For this review, use the dimensioned drawing (mm, ordinates from the lowest corner) and the shaded views. Coordinates: 2 decimals unless noted, no trailing zeros. Write each loop counter-clockwise with the first axis right and the second up, starting at its lowest first coordinate (ties: lowest second). Pieces come first, ordered by that corner, then holes.
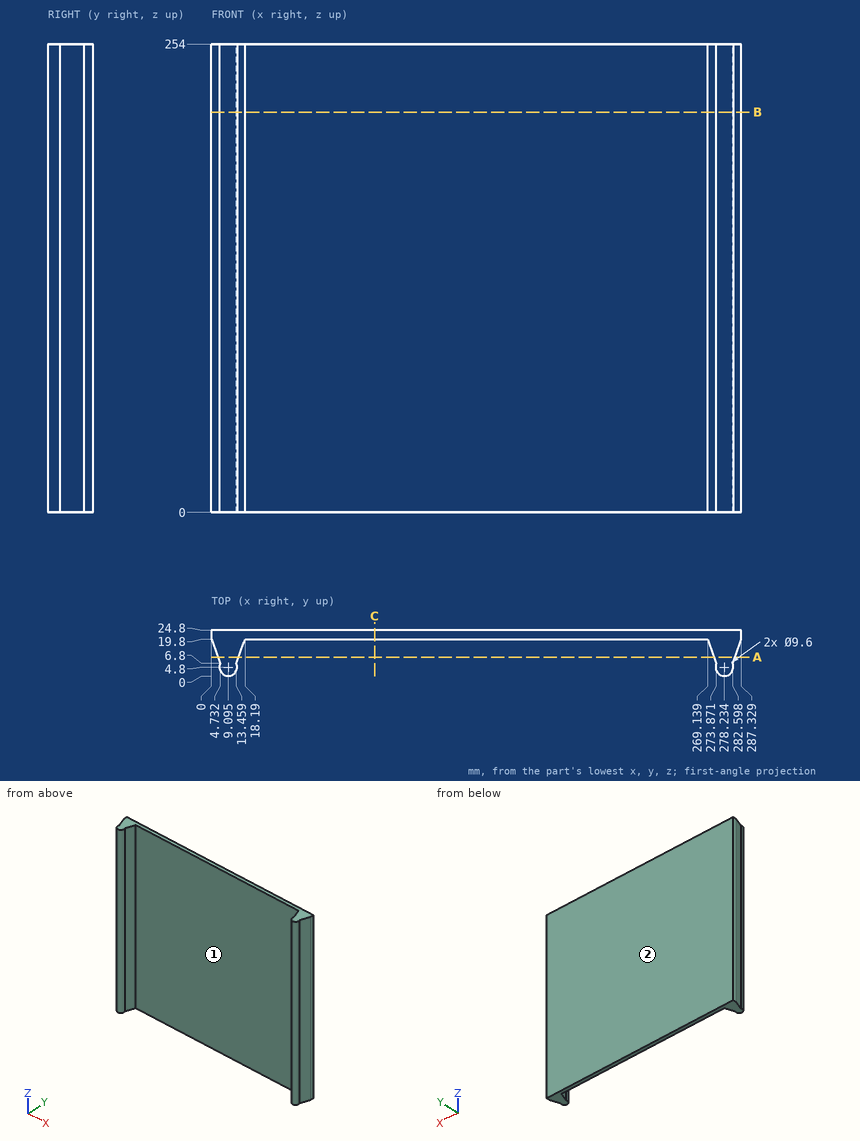
(1) Consider section B-B (z = 217). Give the boundary of the cut face in (x, y) (1 decimal).
(2) Mouldability with a two-part tool opening along X and no side actions: class the marked faces 1 and 2 as +X half, -X half, draft (parallel to the pull), parting line (faces both ways), or undercut.
(3) Consider section C-C (x = 88.5). Give the boundary of the cut face in (y, z), plus the area to 3 significant figures.
(4) Insertion check: pin 1 Ø1.5 at (y, z) = (18.5, 185) entering from +X; pin 2 Ø6 at (y, z) = (7, 61.5) entering from -X; pin 3 Ø10 at (y, z) = (10.5, 155) entering from -X (1 decimal). Each pin has a flat end and moves straight along its axis. Give the tip position at first contact, or say it passes through.
(5) Consider section A-A (y = 10.25). Give the boundary of the cut face in (x, z) (1 decimal), plus the area to 3 significant figures.
(6) Wall thickness on line 1 (X direction, y = 19.75, z = 243); line 2 (Y direction, x = 51.5, z = 50.5); line 3 (X direction, y = 2.25, z = 180): over which ranges is each line inside the solid? List them lowest first.
Results:
1. outline: (0, 19.8) - (4.7, 6.8) arc R4.8 ccw (long way) to (13.5, 6.8) - (18.2, 19.8) - (269.1, 19.8) - (273.9, 6.8) arc R4.8 ccw (long way) to (282.6, 6.8) - (287.3, 19.8) - (287.3, 24.8) - (0, 24.8) - close
2. face 1: undercut
2. face 2: draft
3. outline: (19.8, 0) - (24.8, 0) - (24.8, 254) - (19.8, 254) - close
3. area: 1,270 mm2
4. pin 1: stops at x = 287.13
4. pin 2: stops at x = 3.57
4. pin 3: stops at x = 1.6
5. outline: (3.5, 0) - (14.7, 0) - (14.7, 254) - (3.5, 254) - close; (272.6, 0) - (283.9, 0) - (283.9, 254) - (272.6, 254) - close
5. area: 5,710 mm2
6. line 1: x = 0.02 to 18.17, 269.16 to 287.31
6. line 2: y = 19.8 to 24.8
6. line 3: x = 5.03 to 13.16, 274.17 to 282.3
